Here's how the part is built. I have some questions about the finished solid (model axes, mm). Give positions to 0.01 mm unless a question says otherwise; leave off trailing zeros. Write each loop counter-clockwise with the first axis right and the second up, starting at its lowest first coordinate (ties: lowest second). Pieces come first, ordered by that corner, then holes. Notation, with made-up numbers: M 77,79.5 L 100,79.5 A17 cw 100,111.5 Z; hole C 66,62.25 d2. An arc over 180 degrees is marked long. Answer as CSV lines item,"result". Start each with the question number.
Q1. If I drill on line 1 along Y through (x, z) = (0, 1.1); line 2 along Y through (x, z) = (0, 3.9); line 3 along Y through (x, z) = (-26, 0.35), over which ranges is the centre line in solid material (lowest first)?
Q2. Suppose I cut it at C-C (y = 10). Write out the boundary of the cut face in (x, z).
Q3. Suppose I cut it at A-A (x = 0). Write out the boundary of the cut face in (y, z).
Q4. For pin 1 (1.5 mm diameter, centred on x = -22.5, z = 1.5, fed in from -Y); pin 2 (4.5 mm diameter, centred on x = -24.68, y = 14.25, fed in from -Z); pin 3 (1 mm diameter, centred on x = -7, z = 1, fed in from +Y), each with a flat end and sliding along its axis, tell me the tip position at first contact or that it passes through.
Q5. Suppose I cut it at B-B (z = 3.75). Write out the boundary of the cut face in (x, y), then the cut area to 3 significant figures.
Q6. Suppose I cut it at D-D (x = -19). Write out the boundary of the cut face in (y, z), then the cut area to 3 significant figures.
```python
from build123d import *

# Parameters (mm, degrees)
SKETCH_1_R          = 32
SKETCH_1_R_2        = 24
EXTRUDE_1_DEPTH     = 2
SKETCH_2_R          = 32
SKETCH_2_R_2        = 25
EXTRUDE_2_DEPTH     = 4
SKETCH_3_R          = 1.8
CUT_EXTRUDE_1_DEPTH = 46.650848842
SKETCH_4_R          = 2.85
CUT_EXTRUDE_2_DEPTH = 3
SKETCH_5_R          = 32
SKETCH_5_R_2        = 25
SKETCH_5_R_3        = 1.8
CUT_EXTRUDE_3_DEPTH = 1


with BuildPart() as part:
    # 草图1 → 凸台-拉伸1 (new body)
    with BuildSketch(Plane.XY):
        Circle(SKETCH_1_R)
        Circle(SKETCH_1_R_2, mode=Mode.SUBTRACT)
    extrude(amount=EXTRUDE_1_DEPTH)

    # 草图2 → 凸台-拉伸2 (add)
    with BuildSketch(Plane.XY.offset(2)):
        Circle(SKETCH_2_R)
        Circle(SKETCH_2_R_2, mode=Mode.SUBTRACT)
    extrude(amount=EXTRUDE_2_DEPTH)

    # 草图3 → 切除-拉伸1 (cut, through all)
    with BuildSketch(Plane.XY.offset(6)):
        with Locations((0, 28.5)):
            Circle(SKETCH_3_R)
        with Locations((24.681724008, 14.25)):
            Circle(SKETCH_3_R)
        with Locations((24.681724008, -14.25)):
            Circle(SKETCH_3_R)
        with Locations((0, -28.5)):
            Circle(SKETCH_3_R)
        with Locations((-24.681724008, -14.25)):
            Circle(SKETCH_3_R)
        with Locations((-24.681724008, 14.25)):
            Circle(SKETCH_3_R)
    extrude(amount=-CUT_EXTRUDE_1_DEPTH, mode=Mode.SUBTRACT)

    # 草图4 → 切除-拉伸2 (cut)
    with BuildSketch(Plane(origin=(0, 0, 0), x_dir=(-1, 0, 0), z_dir=(0, 0, -1))):
        with Locations((-24.681724008, -14.25)):
            Circle(SKETCH_4_R)
        with Locations((-24.681724008, 14.25)):
            Circle(SKETCH_4_R)
        with Locations((0, 28.5)):
            Circle(SKETCH_4_R)
        with Locations((24.681724008, 14.25)):
            Circle(SKETCH_4_R)
        with Locations((24.681724008, -14.25)):
            Circle(SKETCH_4_R)
        with Locations((0, -28.5)):
            Circle(SKETCH_4_R)
    extrude(amount=-CUT_EXTRUDE_2_DEPTH, mode=Mode.SUBTRACT)

    # 草图5 → 切除-拉伸3 (cut)
    with BuildSketch(Plane.XY.offset(6)):
        Circle(SKETCH_5_R)
        Circle(SKETCH_5_R_2, mode=Mode.SUBTRACT)
        with Locations((-24.681724008, 14.25)):
            Circle(SKETCH_5_R_3, mode=Mode.SUBTRACT)
        with Locations((0, 28.5)):
            Circle(SKETCH_5_R_3, mode=Mode.SUBTRACT)
        with Locations((24.681724008, 14.25)):
            Circle(SKETCH_5_R_3, mode=Mode.SUBTRACT)
        with Locations((24.681724008, -14.25)):
            Circle(SKETCH_5_R_3, mode=Mode.SUBTRACT)
        with Locations((0, -28.5)):
            Circle(SKETCH_5_R_3, mode=Mode.SUBTRACT)
        with Locations((-24.681724008, -14.25)):
            Circle(SKETCH_5_R_3, mode=Mode.SUBTRACT)
    extrude(amount=-CUT_EXTRUDE_3_DEPTH, mode=Mode.SUBTRACT)


solid = part.part
```
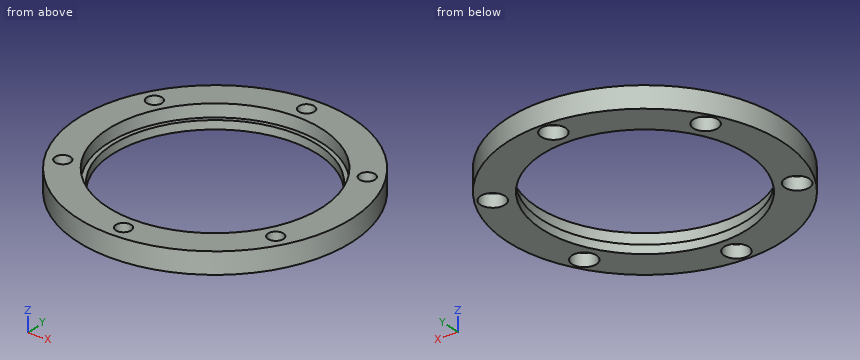
Resolved:
1,line 1,"-32 to -31.35, -25.65 to -24, 24 to 25.65, 31.35 to 32"
1,line 2,"-32 to -30.3, -26.7 to -25, 25 to 26.7, 30.3 to 32"
1,line 3,"-18.65 to -16.78, -11.72 to 11.72, 16.78 to 18.65"
2,outline,"M -30.4,0 L -21.82,0 L -21.82,2 L -22.91,2 L -22.91,5 L -30.4,5 Z; M 21.82,0 L 30.4,0 L 30.4,5 L 22.91,5 L 22.91,2 L 21.82,2 Z"
3,outline,"M -32,0 L -31.35,0 L -31.35,3 L -30.3,3 L -30.3,5 L -32,5 Z; M -26.7,3 L -25.65,3 L -25.65,0 L -24,0 L -24,2 L -25,2 L -25,5 L -26.7,5 Z; M 24,0 L 25.65,0 L 25.65,3 L 26.7,3 L 26.7,5 L 25,5 L 25,2 L 24,2 Z; M 30.3,3 L 31.35,3 L 31.35,0 L 32,0 L 32,5 L 30.3,5 Z"
4,pin 1,"y = -23.47"
4,pin 2,"z = 3"
4,pin 3,"y = 31.33"
5,outline,"C 0,0 d64; hole C -24.68,-14.25 d3.6; hole C -24.68,14.25 d3.6; hole C 0,0 d50; hole C 0,-28.5 d3.6; hole C 0,28.5 d3.6; hole C 24.68,-14.25 d3.6; hole C 24.68,14.25 d3.6"
5,area,"1,190 mm^2"
6,outline,"M -25.75,0 L -14.66,0 L -14.66,2 L -16.25,2 L -16.25,5 L -25.75,5 Z; M 14.66,0 L 25.75,0 L 25.75,5 L 16.25,5 L 16.25,2 L 14.66,2 Z"
6,area,"101 mm^2"
